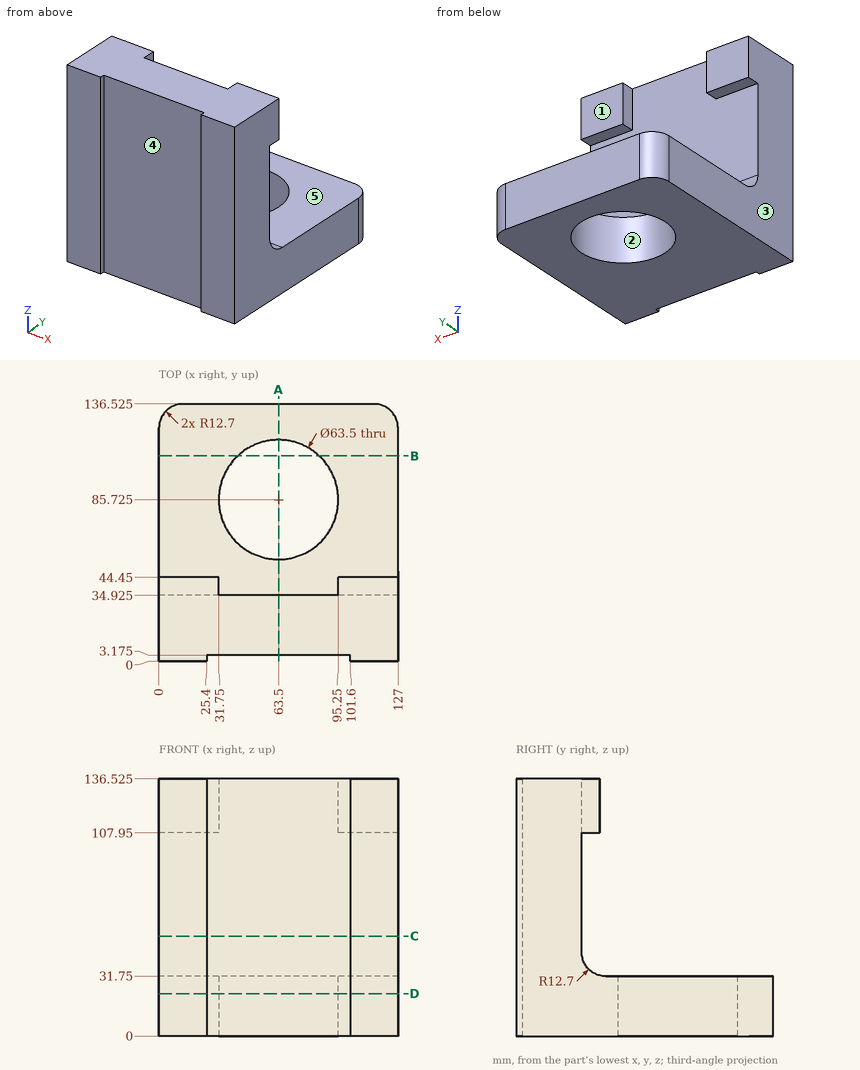
The figure shows three views and two pictorial views of one solid part (mm, origin at its lowest corner). Answer the questions. A direction names the side the tool comes from. Give positions to 0.01 mm unless a question says otherwise; leave off trailing zeros. Write each loop counter-clockwise with the first axis right and the second up, starting at its lowest first coordinate (ties: lowest second). Pieces come first, ordered by that corner, then holes. Notation, with made-up numbers: (27, -29) -> (41, -29) arc R29 ccw to (41, 1) -> close; hole circle Ø3 at (79.5, -34). An arc over 180 degrees is marked (long way). Use one line per item in the form item = value.
1) Section B-B on y = 109 is taken. Write down the section's boundary in (x, z).
Result:
outline = (0, 0) -> (41.91, 0) -> (41.91, 31.75) -> (0, 31.75) -> close; (85.09, 0) -> (127, 0) -> (127, 31.75) -> (85.09, 31.75) -> close
2) A tool of negligible diameter and unlimited length cuts with its end or side. For the marked faces 1 and 2, from which of +Z, -Z, +X, -X, +Y, -Y can it reach the whole face along a straight path? Write none if from no direction.
Result:
face_1 = +Z, +X, -X, +Y
face_2 = +Z, -Z
3) Straight lines are drawn through the part: probe 1 along Y at (x, z) = (23, 60.5) (3 decimals); probe 2 along Y at (x, z) = (63.5, 18) (3 decimals); probe 3 along Z at (x, y) = (16.5, 65). For each, find the intervals that lie inside material, in ascending order.
Result:
probe_1 = 0 to 34.925
probe_2 = 3.175 to 53.975, 117.475 to 136.525
probe_3 = 0 to 31.75
4) For a pull along X with two mould halves and no side action, classify the marked faces 3, 4 and 5 as +X half, -X half, draft (parallel to the pull), parting line (faces both ways), or undercut.
Result:
face_3 = -X half
face_4 = undercut
face_5 = draft
5) Section C-C on z = 53 is taken. Write down the section's boundary in (x, y) (3 decimals), plus the area to 3 significant figures.
Result:
outline = (0, 0) -> (25.4, 0) -> (25.4, 3.175) -> (101.6, 3.175) -> (101.6, 0) -> (127, 0) -> (127, 34.925) -> (0, 34.925) -> close
area = 4,190 mm²
6) Section D-D on z = 22.5 is taken. Write down the section's boundary in (x, y) (3 decimals).
Result:
outline = (0, 0) -> (25.4, 0) -> (25.4, 3.175) -> (101.6, 3.175) -> (101.6, 0) -> (127, 0) -> (127, 123.825) arc R12.7 ccw to (114.3, 136.525) -> (12.7, 136.525) arc R12.7 ccw to (0, 123.825) -> close; hole circle Ø63.5 at (63.5, 85.725)
7) Section A-A on x = 63.5 is taken. Write down the section's boundary in (y, z) (3 decimals), plus the area to 3 significant figures.
Result:
outline = (3.175, 0) -> (53.975, 0) -> (53.975, 31.75) -> (47.625, 31.75) arc R12.7 cw to (34.925, 44.45) -> (34.925, 136.525) -> (3.175, 136.525) -> close; (117.475, 0) -> (136.525, 0) -> (136.525, 31.75) -> (117.475, 31.75) -> close
area = 5,580 mm²
8) Each of these flat-tipped pins is pushed along its axis until it touches: P1, Ø14.5, axis at x = 21.5, z = 116.5, coming from the +Y side; P2, Ø6, axis at x = 90, z = 74.5, coming from the +Y side (3 decimals); P3, Ø1, axis at x = 18.5, y = 79.5, coming from the +Z side. Where does it stop, or does it pass through?
Result:
P1 = 44.45
P2 = 34.925
P3 = 31.75
